from build123d import *

# Parameters (mm, degrees)
SKETCH1_R           = 6
BOSS_EXTRUDE1_DEPTH = 10
M4_TAPPED_HOLE1_D   = 3.3
CIRPATTERN1_COUNT   = 3
BOSS_EXTRUDE2_START = -10
BOSS_EXTRUDE2_DEPTH = 10


with BuildPart() as part:
    # Sketch1 → Boss-Extrude1 (new body)
    with BuildSketch(Plane.XY):
        with BuildLine():
            Line((0, 12), (10, 12))
            ThreePointArc((10, 12), (22, 0), (10, -12))
            Line((10, -12), (0, -12))
            ThreePointArc((0, -12), (-12, 0), (0, 12))
        make_face()
        with Locations((5, 0)):
            Circle(SKETCH1_R, mode=Mode.SUBTRACT)
    extrude(amount=BOSS_EXTRUDE1_DEPTH)

    # M4 Tapped Hole1 (through all)
    with Locations(Plane(origin=(14, 0, 10), x_dir=(1, 0, 0), z_dir=(0, 0, 1))):
        with Locations((0, 0)):
            m4_tapped_hole1 = Hole(M4_TAPPED_HOLE1_D / 2)

    # CirPattern1: M4 Tapped Hole1 ×3 about axis
    cirpattern1_axis = Axis((5, 0, 0), (0, 0, 1))
    for i in range(1, CIRPATTERN1_COUNT):
        add(m4_tapped_hole1.rotate(cirpattern1_axis, i * 360 / CIRPATTERN1_COUNT), mode=Mode.SUBTRACT)

    # Sketch4 → Boss-Extrude2 (add)
    with BuildSketch(Plane.XY.offset(10).offset(BOSS_EXTRUDE2_START)):
        with BuildLine():
            ThreePointArc((9.472135955, 4), (5, 6), (0.527864045, 4))
            Line((0.527864045, 4), (9.472135955, 4))
        make_face()
        with BuildLine():
            Line((9.472135955, -4), (0.527864045, -4))
            ThreePointArc((0.527864045, -4), (5, -6), (9.472135955, -4))
        make_face()
    extrude(amount=BOSS_EXTRUDE2_DEPTH)


solid = part.part
The listing builds one solid part. Answer for the finished solid, in the listing's coordinates (mm). A direction names the side the tool comes from. Coordinates: 2 decimals unless noted, no trailing zeros. Order: outer loops, then holes, each group sorted by start corner. A loop starts at its lowest first (then second) coordinate and runs counter-clockwise, first axis right, second up. Notation, with made-up numbers: M 45,2 L 49,2 A13 ccw 49,12 Z; hole C 52,32 d4. An arc over 180 degrees is marked long. Use CSV: the item, a comma, the result in double quotes.
Q1. Section D-D (x = 17) is taken. Determine the outline of the cut face in (y, z), then the cut area to 3 significant figures.
Here are the results:
outline,"M -9.75,0 L 9.75,0 L 9.75,10 L -9.75,10 Z"
area,"195 mm2"
Q2. Section B-B (y = -9) is taken. Determine the outline of the cut face in (x, z), then the cut area to 3 significant figures.
Here are the results:
outline,"M -7.94,0 L -0.63,0 L -0.63,10 L -7.94,10 Z; M 1.63,0 L 17.94,0 L 17.94,10 L 1.63,10 Z"
area,"236 mm2"
Q3. Section C-C (z = 4.5) is taken. Determine the outline of the cut face in (x, y) (3 decimals), then the cut area to 3 significant figures.
Here are the results:
outline,"M 0,-12 L 10,-12 A12 ccw 10,12 L 0,12 A12 ccw Z; hole C 0.5,-7.794 d3.3; hole C 0.5,7.794 d3.3; hole M 0.528,-4 L 9.472,-4 A6 ccw 9.472,4 L 0.528,4 A6 ccw Z; hole C 14,0 d3.3"
area,"578 mm2"
Q4. Section A-A (x = 7.5) is taken. Determine the outline of the cut face in (y, z), then the cut area to 3 significant figures.
Here are the results:
outline,"M -12,0 L -4,0 L -4,10 L -12,10 Z; M 4,0 L 12,0 L 12,10 L 4,10 Z"
area,"160 mm2"
Q5. Straight lines are drawn through the part: L1, parallel to Y at x = 7, z = 5.75; L2, parallel to Y at x = 0.5, z = 4.5; L3, parallel to Y at x = 1.5, z = 3.25. For each, find the intervals that lie inside material, in ascending order.
Here are the results:
L1,"-12 to -4, 4 to 12"
L2,"-12 to -9.44, -6.14 to -3.97, 3.97 to 6.14, 9.44 to 12"
L3,"-12 to -9.11, -6.48 to -4, 4 to 6.48, 9.11 to 12"
Q6. Given pin 1 Ø3 at (y, z) = (-5.5, 5.5) entering from +X; pin 2 Ø3 at (x, z) = (15, 6) entering from +Y; pin 3 Ø3 at (y, z) = (6, 8.5) entering from -X; pin 4 Ø2 at (x, y) = (0.5, 7.79) entering from +Z, each flat-ended and moving along its own axis, determine where each tip first touches the part or whether it passes through.
Here are the results:
pin 1,"x = 21.31"
pin 2,"y = 11.48"
pin 3,"x = -11.12"
pin 4,"through"
Q7. A tool of negligible diameter and unlimited length cuts with its end or side. For faces 5 (the cylindrical face through (11, 0, 5)), 6 (the flat face through (5, 6, 0)), from which of +Z, -Z, +X, -X, +Y, -Y can it reach the whole face along a straight path? Write none if from no direction.
Here are the results:
face 5,"+Z, -Z"
face 6,"-Z, +X, -X, +Y, -Y"
Q8. Determine the mould class of faces 1 (the cylindrical face through (-1, 0, 5)), 2 (the flat face through (5, -12, 5)), 3 (the cylindrical face through (0.858, -9.405, 4.93)), 4 (the cylindrical face through (-12, 0, 5)) for opening direction Y: pulls with the +Y half, pulls with the -Y half, needs draft (parallel to the pull), parting line crosses it, or undercut.
Here are the results:
face 1,"undercut"
face 2,"pulls with the -Y half"
face 3,"undercut"
face 4,"parting line crosses it"
